```python
from build123d import *

# Parameters (mm, degrees)
SKETCH2_R           = 150
SKETCH2_R_2         = 100
SKETCH2_R_3         = 38.1
SKETCH2_R_4         = 50.8
SKETCH2_R_5         = 63.5
SKETCH2_R_6         = 20
BOSS_EXTRUDE1_DEPTH = 202.5


with BuildPart() as part:
    # Sketch2 → Boss-Extrude1 (new, symmetric)
    with BuildSketch(Plane(origin=(0, 0, 0), x_dir=(0, 0, -1), z_dir=(1, 0, 0))):
        with Locations((169.380920233, 917.544072258)):
            Circle(SKETCH2_R)
        with BuildLine():
            ThreePointArc((148.612903403, 715.363750631), (194.853343441, 714.245445857), (235.644139642, 692.438569744))
            Line((235.644139642, 692.438569744), (224.380920233, 777.991214889))
            ThreePointArc((224.380920233, 777.991214889), (190.549773257, 769.045319194), (155.566499173, 768.1815543))
            Line((155.566499173, 768.1815543), (148.612903403, 715.363750631))
        make_face()
        with Locations((169.380920233, 617.544072258)):
            Circle(SKETCH2_R_2)
        with BuildLine():
            Line((133.64293857, 479.444072258), (156.147736241, 518.423525239))
            ThreePointArc((156.147736241, 518.423525239), (113.74819605, 534.447742616), (82.778379855, 567.544072258))
            Line((82.778379855, 567.544072258), (133.64293857, 479.444072258))
        make_face()
        with BuildLine():
            Line((62.676488117, 356.526574441), (133.64293857, 479.444072258))
            Line((133.64293857, 479.444072258), (82.778379855, 567.544072258))
            ThreePointArc((82.778379855, 567.544072258), (81.231422133, 570.324733162), (79.773717129, 573.15320437))
            Line((79.773717129, 573.15320437), (19.154340526, 443.154531728))
            Line((19.154340526, 443.154531728), (57.677758088, 401.418150827))
            ThreePointArc((57.677758088, 401.418150827), (65.165350074, 389.449758606), (67.780920233, 375.576574441))
            ThreePointArc((67.780920233, 375.576574441), (66.482694215, 365.715568823), (62.676488117, 356.526574441))
        make_face()
        with Locations((29.680920233, 375.576574441)):
            Circle(SKETCH2_R_3)
        with BuildLine():
            Line((57.677758088, 401.418150827), (19.154340526, 443.154531728))
            Line((19.154340526, 443.154531728), (-4.849406453, 391.678330213))
            ThreePointArc((-4.849406453, 391.678330213), (23.816822223, 413.222588234), (57.677758088, 401.418150827))
        make_face()
        with BuildLine():
            Line((-4.849406453, 391.678330213), (19.154340526, 443.154531728))
            Line((19.154340526, 443.154531728), (-157.496365653, 634.538412649))
            ThreePointArc((-157.496365653, 634.538412649), (-147.512909672, 618.580556354), (-144.025482794, 600.082977468))
            ThreePointArc((-144.025482794, 600.082977468), (-174.45020497, 553.548172713), (-229.280917975, 562.753860328))
            Line((-229.280917975, 562.753860328), (3.839343847, 347.579736586))
            ThreePointArc((3.839343847, 347.579736586), (-7.700400772, 368.211329036), (-4.849406453, 391.678330213))
        make_face()
        with Locations((-194.825482794, 600.082977468)):
            Circle(SKETCH2_R_4)
        with BuildLine():
            ThreePointArc((365.001588936, 280.188650866), (440.600513293, 289.717914732), (500.966460612, 243.221069268))
            Line((500.966460612, 243.221069268), (255.983460612, 667.544072258))
            ThreePointArc((255.983460612, 667.544072258), (265.973502862, 643.425976769), (269.380920233, 617.544072258))
            ThreePointArc((269.380920233, 617.544072258), (235.247002555, 542.300074494), (156.147736241, 518.423525239))
            Line((156.147736241, 518.423525239), (133.64293857, 479.444072258))
            Line((133.64293857, 479.444072258), (277.392641257, 230.462283632))
            Line((277.392641257, 230.462283632), (365.001588936, 280.188650866))
        make_face()
        with BuildLine():
            ThreePointArc((327.761379855, 143.221069268), (317.867074769, 219.457662328), (365.001588936, 280.188650866))
            Line((365.001588936, 280.188650866), (277.392641257, 230.462283632))
            Line((277.392641257, 230.462283632), (327.761379855, 143.221069268))
        make_face()
        with Locations((414.363920233, 193.221069268)):
            Circle(SKETCH2_R_2)
        with BuildLine():
            Line((306.939939608, 46.519626158), (449.255457905, 99.505645783))
            ThreePointArc((449.255457905, 99.505645783), (380.507362333, 99.126789489), (327.761379855, 143.221069268))
            Line((327.761379855, 143.221069268), (277.392641257, 230.462283632))
            Line((277.392641257, 230.462283632), (-31.345080373, 55.224414315))
            ThreePointArc((-31.345080373, 55.224414315), (-14.497190191, 61.822985018), (3.527777778, 63.401930443))
            Line((3.527777778, 63.401930443), (306.939939608, 46.519626158))
        make_face()
        Circle(SKETCH2_R_5)
        with BuildLine():
            Line((22.156126422, -59.509293913), (306.939939608, 46.519626158))
            Line((306.939939608, 46.519626158), (3.527777778, 63.401930443))
            ThreePointArc((3.527777778, 63.401930443), (46.131680486, 43.636201204), (63.5, 0))
            ThreePointArc((63.5, 0), (52.149611829, -36.23076022), (22.156126422, -59.509293913))
        make_face()
        with BuildLine():
            Line((459.316666667, 38.041158266), (306.939939608, 46.519626158))
            Line((306.939939608, 46.519626158), (22.156126422, -59.509293913))
            ThreePointArc((22.156126422, -59.509293913), (12.988606104, -62.157430059), (3.527777778, -63.401930443))
            Line((3.527777778, -63.401930443), (437.66530145, -39.245872453))
            Line((437.66530145, -39.245872453), (425.573363507, -21.24537277))
            ThreePointArc((425.573363507, -21.24537277), (424.087573777, 18.846146281), (459.316666667, 38.041158266))
        make_face()
        with Locations((457.2, 0)):
            Circle(SKETCH2_R_3)
        with BuildLine():
            Line((608.509239254, -222.167513639), (491.412350778, 16.766784254))
            ThreePointArc((491.412350778, 16.766784254), (494.315364505, 8.605795586), (495.3, 0))
            ThreePointArc((495.3, 0), (484.879008291, -26.181720723), (459.316666667, -38.041158266))
            Line((459.316666667, -38.041158266), (437.66530145, -39.245872453))
            Line((437.66530145, -39.245872453), (573.94809108, -242.12140184))
            ThreePointArc((573.94809108, -242.12140184), (580.55, -213.648467114), (608.509239254, -222.167513639))
        make_face()
        with Locations((590.55, -230.968975189)):
            Circle(SKETCH2_R_6)
        with BuildLine():
            ThreePointArc((459.316666667, -38.041158266), (440.222538989, -34.108295437), (425.573363507, -21.24537277))
            Line((425.573363507, -21.24537277), (437.66530145, -39.245872453))
            Line((437.66530145, -39.245872453), (459.316666667, -38.041158266))
        make_face()
    extrude(amount=BOSS_EXTRUDE1_DEPTH, both=True)


solid = part.part
```
Here's how the part is built. I have some questions about the finished solid (model axes, mm). A direction names the side the tool comes from. Give positions to 0.01 mm unless a question says otherwise; leave off trailing zeros. Order: outer loops, then holes, each group sorted by start corner. A loop starts at its lowest first (then second) coordinate and runs counter-clockwise, first axis right, second up. Notation, with made-up numbers: M -35,16.25 L 16,16.25 A23 ccw 16,31.25 Z; hole C 46,45 d1. An arc over 180 degrees is marked long. Use a Markdown table: item, result. Add a question column.
1. I need wall thicknesses on probe 1 along Y at (x, z) = (-149, -135.5); probe 2 along Y at (x, z) = (-19.5, -355); probe 3 along Y at (x, z) = (181.5, -186). Which ranges of each line are inside material? Lowest first, please. Write a range as from..to.
2. On a 3-axis mill with a long thin cutter (end or side, diameter ignored), from which of +Z, -Z, +X, -X, +Y, -Y can I reach the whole of each face in a straight line? I mean faces 5 (the flat face through (2.835, -51.493, -217.558)), 6 (the cylindrical face through (2.835, 31.6, -478.485)), 7 (the flat face through (2.84, 356.7, -204.51)). Say none if no direction works.
3. Suppose I cut it at B-B (y = 543). List the corners of the cut face in (x, z) for me, and give its area (3 significant figures).
4. Suppose I cut it at C-C (z = -590.55). List the corners of the cut face in (x, y) for me, and give its area (3 significant figures).
5. If we mould it in two halves opening along Z, with no side actions, what happens to faces 1 (the cylindrical face through (2.84, 1066.78, -154.27)), 2 (the cylindrical face through (2.84, 337.84, -34.94)), 3 (the flat face through (2.84, 417.12, -97.66)), 4 (the flat face through (2.84, 452.41, -380.19))? For each: +Z half, -Z half, draft (parallel to the pull), parting line (faces both ways), or undercut.
6. For pin 1 Ø1 at (x, y) = (-8.5, 816.5) entering from +Z; pin 2 Ø3 at (x, z) = (-21, 135.5) entering from +Y; pin 3 Ø1 at (x, y) = (111, 807) entering from +Z, each with a flat end and sliding along its axis, tell me the tip position at first contact or that it passes through.
7. Suppose I cut it at A-A (x = 56). List the corners of the cut face in (y, z) for me.
8. Suppose I cut it at D-D (y = 157.5). List the corners of the cut face in (x, z) for me, and give its area (3 significant figures).
Results list:
| question | item | result |
|---|---|---|
| 1 | probe 1 | y = -56.06..149.92, 476.23..711.63, 771.42..1063.67 |
| 1 | probe 2 | y = -43.85..43.85, 64.41..496.04 |
| 1 | probe 3 | y = -53.25..178.59, 388.76..1066.62 |
| 2 | face 5 | +X, -X, -Y |
| 2 | face 6 | -Z, +X, -X |
| 2 | face 7 | +X, -X |
| 3 | outline | M -202.5,-327.89 L 202.5,-327.89 L 202.5,-65.71 L -202.5,-65.71 Z; M -202.5,73 L 202.5,73 L 202.5,207.88 L -202.5,207.88 Z |
| 3 | area | 161,000 mm² |
| 4 | outline | M -202.5,-250.97 L 202.5,-250.97 L 202.5,-185.52 L -202.5,-185.52 Z |
| 4 | area | 26,500 mm² |
| 5 | face 1 | parting line |
| 5 | face 2 | undercut |
| 5 | face 3 | undercut |
| 5 | face 4 | -Z half |
| 6 | pin 1 | stops at z = -58.07 |
| 6 | pin 2 | stops at y = 612.33 |
| 6 | pin 3 | stops at z = -67.45 |
| 7 | outline | M -242.12,-573.95 A20 ccw -222.17,-608.51 L 16.77,-491.41 A38.1 ccw 38.04,-459.32 L 46.52,-306.94 L 99.51,-449.26 A100 ccw 243.22,-500.97 L 667.54,-255.98 A100 ccw 692.44,-235.64 L 777.99,-224.38 A150 ccw long 768.18,-155.57 L 715.36,-148.61 A100 ccw 573.15,-79.77 L 443.15,-19.15 L 634.54,157.5 A50.8 ccw long 562.75,229.28 L 347.58,-3.84 A38.1 ccw 356.53,-62.68 L 479.44,-133.64 L 230.46,-277.39 L 55.22,31.35 A63.5 ccw -63.4,-3.53 L -39.25,-437.67 Z |
| 8 | outline | M -202.5,-507.77 L 202.5,-507.77 L 202.5,-148.85 L -202.5,-148.85 Z |
| 8 | area | 145,000 mm² |
